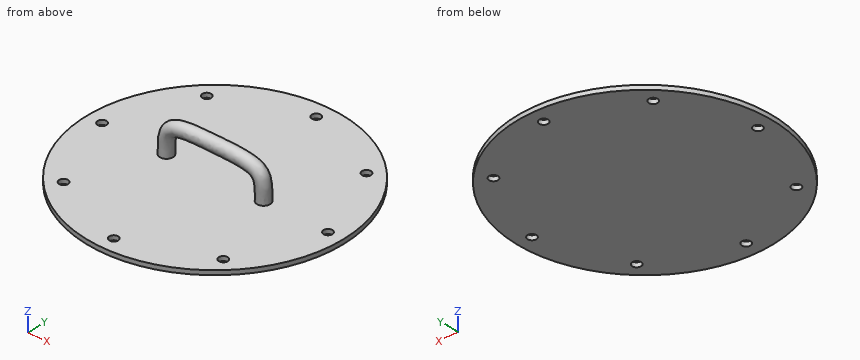
Autodesk Inventor part; units mm, degrees
ref_plane "YZ Plane" through (0, 0, 0) normal (1, 0, 0) x (0, 1, 0)
ref_plane "XZ Plane" through (0, 0, 0) normal (0, 1, 0) x (-1, 0, 0)
ref_plane "XY Plane" through (0, 0, 0) normal (0, 0, 1) x (1, 0, 0)
sketch "草图1" plane through (0, 0, 0) normal (0, 0, 1) x (1, 0, 0)
  circle A0 centre (0, 0) radius 290
  dimension "d0" = 580
extrude "拉伸1" add sketch "草图1" along normal blind 10
sketch "草图2" plane through (0, 0, 0) normal (0, 0, 1) x (1, 0, 0)
  line L0 (0, 0) -> (255.65, 0)
  circle A0 centre (0, 0) radius 255.65
  dimension "d4" = 255.65
hole "孔1" at (255.65, 0, 0) direction (0, 0, 1) diameter 20 end through all
pattern_circular "环形阵列1" count 8 over 360 about axis through (0, 0, -10) along (0, 0, 1) of "孔1"
sketch "草图3" plane through (0, 0, 10) normal (0, 0, 1) x (1, 0, 0)
  circle A0 centre (0, 0) radius 290
  circle A1 centre (-110, 0) radius 15
  circle A2 centre (110, 0) radius 15
  dimension "d15" = 30
  dimension "d16" = 110
  dimension "d18" = 30
  dimension "d19" = 110
sketch "草图4" plane through (0, 0, 0) normal (0, 1, 0) x (-1, 0, 0)
  line L0 (110, 10) -> (110, 52.7861) construction
  line L1 (-110, 52.7861) -> (-110, 10) construction
  spline S0 degree 4 poles (110, 10) (110, 52.7861) (110, 76.933) (17.246, 76.933) (-17.246, 76.933) (-110, 76.933) (-110, 52.7861) (-110, 10) knots 1 1 1 1 1 1.296402 1.477939 1.714323 2 2 2 2 2
  line L2 (110, 52.7861) -> (110, 76.933) construction
  line L3 (-110, 76.933) -> (-110, 52.7861) construction
  line L4 (110, 76.933) -> (17.246, 76.933) construction
  line L5 (17.246, 76.933) -> (-17.246, 76.933) construction
  line L6 (-17.246, 76.933) -> (-110, 76.933) construction
  line L7 (0, -18.6745) -> (0, 112.0473)
  point P0 (0, 0)
sweep "扫掠2" add profiles "草图3" path "草图4" path curves S0 contours A1
properties part number "人孔法兰"
For this review, take the finished solid that the model builds, in its own axes (mm). Round coordinates to 2 decimals unless told otherwise and drop trailing zeros. Write each loop counter-clockwise with the first axis right and the second up, starting at its lowest first coordinate (ties: lowest second). Pieces come first, ordered by that corner, then holes.
1) Take a section at C-C on y = 0. State how many separate pieces and enclosed holes the cut face has, then the cut area to 3 significant figures.
Answer below:
separate pieces: 3
enclosed holes: 1
area: 14,900 mm2
2) For line 1 along Y through (x, z) = (0, 5); line 2 along Z through (x, y) = (-210, -64); line 3 along Y through (x, z) = (255.65, 5.5), list the stretches that pass through material, from the lowest coordinate up.
Answer below:
line 1: y = -290 to -265.65, -245.65 to 245.65, 265.65 to 290
line 2: z = 0 to 10
line 3: y = -136.91 to -10, 10 to 136.91
3) Insertion check: pin 1 Ø2 at (x, z) = (-108.5, 57) entering from +Y; pin 2 Ø12 at (x, y) = (0, -255.65) entering from -Z; pin 3 Ø4 at (x, z) = (-15.5, 67.5) entering from -Y. Each pin has a flat end and moves straight along its axis. Give the tip position at first contact, or say it passes through.
Answer below:
pin 1: stops at y = 14.8
pin 2: passes through
pin 3: stops at y = -13.03
4) Take a section at A-A on y = -255.65. Give the boundary of the cut face in (x, z), then the cut area to 3 significant figures.
Answer below:
outline: (-136.91, 0) - (-10, 0) - (-10, 10) - (-136.91, 10) - close; (10, 0) - (136.91, 0) - (136.91, 10) - (10, 10) - close
area: 2,540 mm2
